Check sheet for the modelled part. Datum: model origin and axes. Units: mm. A direction names the side the tool comes from. Give positions to 0.01 mm unless a question says otherwise; leave off trailing zeros. Order: outer loops, then holes, each group sorted by start corner. A loop starts at its lowest first (then second) coordinate and runs counter-clockwise, first axis right, second up.
Item 1: Sectioned sample at A-A on y = -25. Record the boundary of the cut face in (x, z), and give its area (3 significant figures).
Item 2: Sectioned sample at B-B on x = 44.5. Record the boundary of the cut face in (y, z).
Item 3: Gauge pin test, flat ends, axial feed: P1, Ø1.5, axis at y = -83.5, z = -5.5, coming from the +X side; P2, Ø2, axis at x = 179.5, z = -7.5, coming from the -Y side; P3, Ø4, axis at x = 76, z = -8.5, coming from the -Y side. Record the tip position at first contact, or that the pin passes through.
Item 4: Material ranges on line 1 along Y through (x, z) = (151, -7.5); line 2 along X through (y, z) = (-60, -5); line 3 along Y through (x, z) = (142, -2.5), recorded low to high.
Item 5: Access from +Z, -Z, +X, -X, +Y, -Y to the whole of each face (thin tool, end or side, straight path). Record for faces 4 (the flat face through (269.373, -117.007, -5.035)), 5 (the flat face through (267, -120, -2.5)), 6 (the flat face through (-4, -19.5, -5)), 7 (the flat face through (-4, -7, -4.2)).
Item 6: Release check for a two-part mould opening along Y. For faces 1 (the flat face through (267, -120, -7.5)), 2 (the cylindrical face through (147.93, -29.85, -4.93)), 3 (the flat face through (263, -118.5, -1.6)) record: released by +Y, released by -Y, zero draft, split by the parting line, or undercut.
Autodesk Inventor part; units mm, degrees
ref_plane "YZ Plane" through (0, 0, 0) normal (1, 0, 0) x (0, 1, 0)
ref_plane "XZ Plane" through (0, 0, 0) normal (0, 1, 0) x (-1, 0, 0)
ref_plane "XY Plane" through (0, 0, 0) normal (0, 0, 1) x (1, 0, 0)
sketch "Sketch1" plane through (0, 0, 0) normal (0, 0, 1) x (1, 0, 0)
  arc A0 (381.5, -381.5) -> (0, 0) centre (0, -381.5) ccw
  line L0 (-227, 0) -> (0, 0)
  line L1 (381.5, -381.5) -> (381.5, -681.5)
  line L2 (-227, -19.5) -> (0, -19.5)
  arc A1 (362, -381.5) -> (0, -19.5) centre (0, -381.5) ccw
  line L3 (362, -381.5) -> (362, -681.5)
  line L4 (-8, 0) -> (-8, -19.5)
  line L5 (381.5, -389.5) -> (362, -389.5)
  line L6 (269.7612, -111.7388) -> (255.9727, -125.5273)
  dimension "d0" = 19.5
  dimension "d1" = 8
  dimension "d2" = 8
extrude "Extrusion1" add sketch "Sketch1" against normal blind 10 contours L6 A1 L2 L4 L0 A0
sketch "Sketch2" plane through (-8, -19.5, 0) normal (-1, 0, 0) x (0, 0, 1)
  line L0 (0, 19.5) -> (0, 0)
  line L1 (0, 19.5) -> (-10, 19.5)
  line L2 (-10, 0) -> (-10, 19.5)
  line L3 (0, 0) -> (-10, 0)
  line L4 (-1.2, 14.5) -> (-4.2, 14.5)
  line L5 (-4.2, 14.5) -> (-4.2, 9.5)
  line L6 (-4.2, 9.5) -> (-1.2, 9.5)
  line L7 (-1.2, 9.5) -> (-1.2, 14.5)
  line L8 (-1.2, 14.5) -> (-4.2, 9.5) construction
  line L9 (-4.2, 14.5) -> (-1.2, 9.5) construction
  point P0 (0, 19.5)
  point P1 (-2.7, 12)
  dimension "d5" = 3
  dimension "d6" = 5
  dimension "d7" = 1.2
  dimension "d8" = 5
extrude "Extrusion2" cut sketch "Sketch2" against normal blind 7.1 contours L7 L6 L5 L4
sketch "Sketch3" plane through (255.9727, -125.5273, 0) normal (0.7071, -0.7071, 0) x (-0.7071, -0.7071, 0)
  line L0 (0, 0) -> (-19.5, 0)
  line L1 (0, 0) -> (0, 10)
  line L2 (-19.5, 10) -> (0, 10)
  line L3 (-19.5, 0) -> (-19.5, 10)
  line L4 (-15.5, 2.5) -> (-7.5, 2.5)
  line L5 (-7.5, 2.5) -> (-7.5, 7.5)
  line L6 (-7.5, 7.5) -> (-15.5, 7.5)
  line L7 (-15.5, 7.5) -> (-15.5, 2.5)
  line L8 (-15.5, 2.5) -> (-7.5, 7.5) construction
  line L9 (-7.5, 2.5) -> (-15.5, 7.5) construction
  point P0 (92.2388, 0)
  point P1 (-11.5, 5)
  point P2 (-15.5, 5)
  point P3 (-19.5, 5)
  dimension "d11" = 8
  dimension "d12" = 5
  dimension "d13" = 4
extrude "Extrusion3" add sketch "Sketch3" along normal blind 7 contours L7 L6 L5 L4
properties part number "SEPARADOR_3"
Report:
1. outline: (62.86, -10) - (135.83, -10) - (135.83, 0) - (62.86, 0) - close
1. area: 730 mm2
2. outline: (-22.25, -10) - (-2.6, -10) - (-2.6, 0) - (-22.25, 0) - close
3. P1: stops at x = 239.13
3. P2: stops at y = -67.71
3. P3: stops at y = -28
4. line 1: y = -52.5 to -31.16
4. line 2: x = 166.38 to 205.38
4. line 3: y = -48.51 to -27.41
5. face 4: +Z, -Z, +X
5. face 5: +Z, +X, -Y
5. face 6: +Z, -Z, -X, -Y
5. face 7: -X
6. face 1: zero draft
6. face 2: released by +Y
6. face 3: undercut
